Autodesk Inventor part; units mm, degrees
ref_plane "YZ Plane" through (0, 0, 0) normal (1, 0, 0) x (0, 1, 0)
ref_plane "XZ Plane" through (0, 0, 0) normal (0, 1, 0) x (-1, 0, 0)
ref_plane "XY Plane" through (0, 0, 0) normal (0, 0, 1) x (1, 0, 0)
sketch "Sketch1" plane through (0, 0, 0) normal (0, 1, 0) x (-1, 0, 0)
  circle A0 centre (0, 0) radius 6
  circle A1 centre (0, 0) radius 7.5
  dimension "d0" = 12
  dimension "d1" = 15
extrude "Extrusion1" add sketch "Sketch1" along normal blind 3.5
sketch "Sketch2" plane through (0, 0, 0) normal (0, -1, 0) x (1, 0, 0)
  circle A0 centre (0, 0) radius 4.5
  circle A1 centre (0, 0) radius 8.25
  dimension "d4" = 9
  dimension "d5" = 16.5
extrude "Extrusion2" add sketch "Sketch2" along normal blind 2
sketch "Sketch3" plane through (0, -2, 0) normal (0, -1, 0) x (1, 0, 0)
  circle A0 centre (0, 0) radius 6.75
  circle A1 centre (0, 0) radius 8.25
  circle A2 centre (0, 0) radius 8.25
  dimension "d8" = 13.5
  dimension "d9" = 16.5
extrude "Extrusion3" add sketch "Sketch3" along normal blind 11
sketch "Sketch4" plane through (0, -13, 0) normal (0, -1, 0) x (1, 0, 0)
  point P0 (0, 0)
sketch "Sketch9" plane through (0, -2, 0) normal (0, -1, 0) x (1, 0, 0)
  circle A0 centre (0, 0) radius 6.45
  circle A1 centre (0, 0) radius 6.75
  dimension "d54" = 12.9
  dimension "d55" = 13.5
extrude "Extrusion4" add sketch "Sketch9" along normal blind 2
thread "Thread4"
thread "Thread5"
equation "\"d25\" = 60deg"
equation "\"Sketch5_Pitch\" = 0.5"
equation "\"d43\" = 60deg"
equation "\"Sketch7_Pitch\" = 0.5"
properties part number "holder2"
Source: CAD feature listing. Evaluate the final solid. Frame: model axes, mm. A direction names the side the tool comes from. Round coordinates to 2 decimals unless told otherwise and drop trailing zeros. Loops run counter-clockwise (first coordinate to the right, second up) from the corner with the lowest first, then second, coordinate; pieces in that order, holes last. Notation, with made-up numbers: M 16.25,5.25 L 42.25,5.25 A17 cw 42.25,24.25 Z; hole C 20,38 d10. An arc over 180 degrees is marked long. Use a Markdown table: item, result. Add a question column.
1. Section query D-D on x = 5.5. Return the cut outline in (y, z), then the cut area to 3 significant figures.
2. Section query B-B on z = 0. Return the cut outline in (x, y), then the cut area to 3 significant figures.
3. Section query A-A on x = 0. Return the cut outline in (y, z).
4. Line query: line 1 (Z direction, x = 0, y = -3.5); line 2 (Y direction, x = -6, z = -1.25); line 3 (Z direction, x = 0, y = -0.55). Output: solid intervals per line, ascending.
5. Mould query, pull axis Z, two halves, no side actions, for faces 4 (the cylindrical face through (7.62, -6.41, 3.16)), 5 (the flat face through (3, -2, -4)), 6 (the flat face through (-2, 3.5, 6)). Classes: pulls with the +Z half, pulls with the -Z half, needs draft (parallel to the pull), parting line crosses it, or undercut.
6. Reachability of faces 1 (the cylindrical face through (-1.46, -8.44, 6.59)), 2 (the cylindrical face through (-0.59, -0.99, -4.46)), 3 (the flat face through (-1.4, 0, 4.5)) from +Z, -Z, +X, -X, +Y, -Y: full face, straight path, thin tool, end or side. Return the list, or none.
7. Contact query for flat-ended pins moving along their axis: P1, Ø6, axis at x = 4, z = 1, coming from the +Y side; P2, Ø5, axis at y = -3, z = -6.5, coming from the +X side; P3, Ø1.5, axis at x = 2.5, y = -8.5, coming from the +Z side; P4, Ø1, axis at y = -11, z = 1, coming from the +X side. Output: stop coordinate, or through.
8. Section query C-C on y = -1. Return the cut outline in (x, z).
Reported:
| question | item | result |
|---|---|---|
| 1 | outline | M -13,-6.15 L 0,-6.15 L 0,-5.1 L 3.5,-5.1 L 3.5,-2.4 L 0,-2.4 L 0,2.4 L 3.5,2.4 L 3.5,5.1 L 0,5.1 L 0,6.15 L -13,6.15 L -13,3.91 L -4,3.91 L -4,3.37 L -2,3.37 L -2,-3.37 L -4,-3.37 L -4,-3.91 L -13,-3.91 Z |
| 1 | area | 94.9 mm² |
| 2 | outline | M -8.25,-13 L -6.75,-13 L -6.75,-4 L -6.45,-4 L -6.45,-2 L -4.5,-2 L -4.5,0 L -6,0 L -6,3.5 L -7.5,3.5 L -7.5,0 L -8.25,0 Z; M 4.5,-2 L 6.45,-2 L 6.45,-4 L 6.75,-4 L 6.75,-13 L 8.25,-13 L 8.25,0 L 7.5,0 L 7.5,3.5 L 6,3.5 L 6,0 L 4.5,0 Z |
| 2 | area | 59.7 mm² |
| 3 | outline | M -13,-8.25 L 0,-8.25 L 0,-7.5 L 3.5,-7.5 L 3.5,-6 L 0,-6 L 0,-4.5 L -2,-4.5 L -2,-6.45 L -4,-6.45 L -4,-6.75 L -13,-6.75 Z; M -13,6.75 L -4,6.75 L -4,6.45 L -2,6.45 L -2,4.5 L 0,4.5 L 0,6 L 3.5,6 L 3.5,7.5 L 0,7.5 L 0,8.25 L -13,8.25 Z |
| 4 | line 1 | z = -8.25 to -6.45, 6.45 to 8.25 |
| 4 | line 2 | y = -2 to 3.5 |
| 4 | line 3 | z = -8.25 to -4.5, 4.5 to 8.25 |
| 5 | face 4 | parting line crosses it |
| 5 | face 5 | undercut |
| 5 | face 6 | needs draft |
| 6 | face 1 | -Y |
| 6 | face 2 | +Y, -Y |
| 6 | face 3 | +Y |
| 7 | P1 | stops at y = 3.5 |
| 7 | P2 | stops at x = 7.22 |
| 7 | P3 | stops at z = 8.06 |
| 7 | P4 | stops at x = 8.23 |
| 8 | outline | C 0,0 d16.5; hole C 0,0 d9 |
